Read the model definition and answer for the solid it produces. Units are mm, in the model's axes. A direction names the side the tool comes from. Coordinates: 2 decimals unless noted, no trailing zeros. Write each loop counter-clockwise with the first axis right and the second up, starting at its lowest first coordinate (ties: lowest second). Pieces come first, ordered by that corner, then holes.
(1) Given pin 1 (8 mm diameter, centred on y = 24, z = -23.74, fed in from -X); pin 2 (1.9 mm diameter, centred on x = -8.5, z = -22, fed in from +Y); pin 3 (1.9 mm diameter, centred on x = -7, z = -15, fed in from -Y), each flat-ended and moving along its own axis, determine where each tip first touches the part or whether it passes through.
(2) The mould has two halves that part along Z. Classify faces 4 (the cylindrical face through (-27.285, -1.521, -21.97)), 5 (the flat face through (-55, 71, -31.213)), 6 (the flat face through (-65.2, 116, -16)): +Z half, -Z half, draft (parallel to the pull), parting line (faces both ways), or undercut.
(3) Section C-C on x = -24.5 is taken. Write down the section's boundary in (y, z), then the cut area to 3 significant figures.
(4) Section B-B on x = -33.5 is taken. Write down the section's boundary in (y, z).
(5) Section A-A on y = 112 is taken. Write down the section's boundary in (x, z).
(6) Find the intervals of material crossed by probe 1 along X at (y, z) = (103, -13); probe 2 along X at (y, z) = (8.5, -20); probe 3 along Y at (x, z) = (-12.5, -22), in increasing order.
(7) Which of the six approach directions +Z, -Z, +X, -X, +Y, -Y give full straight-line access (tool end or side, diameter ignored) to faces 1 (the flat face through (-55.6, 41, -16)), 2 (the cylindrical face through (-54.079, 21.793, -21.712)), 3 (the flat face through (-34, 0, -13))?
from build123d import *

# Parameters (mm, degrees)
SKETCH_1_W                       = 44.2
SKETCH_1_H                       = 30
SM_BASE_FLANGE_1_DEPTH           = 3
SM_EDGE_FLANGE_1_STRIP_W         = 13.4732
SM_EDGE_FLANGE_1_STRIP_H         = 3
SM_EDGE_FLANGE_1_STRIP_CUT_DEPTH = 30
SM_EDGE_FLANGE_1_DEPTH           = 30
SM_EDGE_FLANGE_2_STRIP_W         = 13.4732
SM_EDGE_FLANGE_2_STRIP_H         = 3
SM_EDGE_FLANGE_2_STRIP_CUT_DEPTH = 30
SM_EDGE_FLANGE_2_DEPTH           = 30
SM_EDGE_FLANGE_3_STRIP_W         = 13.4732
SM_EDGE_FLANGE_3_STRIP_H         = 3
SM_EDGE_FLANGE_3_STRIP_CUT_DEPTH = 30
SM_EDGE_FLANGE_3_DEPTH           = 30
SM_EDGE_FLANGE_4_STRIP_W         = 13.4732
SM_EDGE_FLANGE_4_STRIP_H         = 3
SM_EDGE_FLANGE_4_STRIP_CUT_DEPTH = 30
SM_EDGE_FLANGE_4_DEPTH           = 30
SM_EDGE_FLANGE_5_STRIP_W         = 13.4732
SM_EDGE_FLANGE_5_STRIP_H         = 3
SM_EDGE_FLANGE_5_STRIP_CUT_DEPTH = 30
SM_EDGE_FLANGE_5_DEPTH           = 30
SM_EDGE_FLANGE_6_STRIP_W         = 13.4732
SM_EDGE_FLANGE_6_STRIP_H         = 3
SM_EDGE_FLANGE_6_STRIP_CUT_DEPTH = 30
SM_EDGE_FLANGE_6_DEPTH           = 30
SKETCH_20_R                      = 6
SKETCH_20_R_2                    = 1.05
CUT_EXTRUDE_1_DEPTH              = 100
SKETCH_21_R                      = 3
SKETCH_21_R_2                    = 1.5
CUT_EXTRUDE_2_DEPTH              = 10
SKETCH_22_R                      = 3
CUT_EXTRUDE_3_DEPTH              = 66


# Sheet-metal steps are written as plain solids
with BuildPart() as part:
    # Sketch 1 → 基体-法兰1 (new body)
    with BuildSketch(Plane(origin=(0, 0, 0), x_dir=(1, 0, 0), z_dir=(0, 1, 0))):
        with Locations((-33.5, 16.21342484)):
            Rectangle(SKETCH_1_W, SKETCH_1_H)
    extrude(amount=-SM_BASE_FLANGE_1_DEPTH)

    # 边线-法兰1 strip (across the edge) → 边线-法兰1 strip cut (cut)
    with BuildSketch(Plane(origin=(-55.6, 0, -31.21342484), x_dir=(1, 0, 0), z_dir=(0, 0, 1))):
        with Locations((-3, -1.5)):
            Rectangle(SM_EDGE_FLANGE_1_STRIP_W, SM_EDGE_FLANGE_1_STRIP_H)
    extrude(amount=SM_EDGE_FLANGE_1_STRIP_CUT_DEPTH, mode=Mode.SUBTRACT)

    # 边线-法兰1 section (across the edge) → 边线-法兰1 (add)
    with BuildSketch(Plane(origin=(-55.6, 0, -31.21342484), x_dir=(1, 0, 0), z_dir=(0, 0, 1))):
        with BuildLine():
            Line((0, 0.7366), (0, 87))
            Line((0, 87), (3, 87))
            Line((3, 87), (3, 0.7366))
            ThreePointArc((3, 0.7366), (3.215745145, 0.215745145), (3.7366, 0))
            Line((3.7366, 0), (3.7366, -3))
            ThreePointArc((3.7366, -3), (1.094424801, -1.905575199), (0, 0.7366))
        make_face()
    extrude(amount=SM_EDGE_FLANGE_1_DEPTH)

    # 边线-法兰2 strip (across the edge) → 边线-法兰2 strip cut (cut)
    with BuildSketch(Plane(origin=(-11.4, 0, -1.21342484), x_dir=(-1, 0, 0), z_dir=(0, 0, -1))):
        with Locations((-3, -1.5)):
            Rectangle(SM_EDGE_FLANGE_2_STRIP_W, SM_EDGE_FLANGE_2_STRIP_H)
    extrude(amount=SM_EDGE_FLANGE_2_STRIP_CUT_DEPTH, mode=Mode.SUBTRACT)

    # 边线-法兰2 section (across the edge) → 边线-法兰2 (add)
    with BuildSketch(Plane(origin=(-11.4, 0, -1.21342484), x_dir=(-1, 0, 0), z_dir=(0, 0, -1))):
        with BuildLine():
            Line((0, 0.7366), (0, 87))
            Line((0, 87), (3, 87))
            Line((3, 87), (3, 0.7366))
            ThreePointArc((3, 0.7366), (3.215745145, 0.215745145), (3.7366, 0))
            Line((3.7366, 0), (3.7366, -3))
            ThreePointArc((3.7366, -3), (1.094424801, -1.905575199), (0, 0.7366))
        make_face()
    extrude(amount=SM_EDGE_FLANGE_2_DEPTH)

    # 边线-法兰3 strip (across the edge) → 边线-法兰3 strip cut (cut)
    with BuildSketch(Plane(origin=(-11.4, 87, -31.21342484), x_dir=(0, -1, 0), z_dir=(0, 0, 1))):
        with Locations((-3, -1.5)):
            Rectangle(SM_EDGE_FLANGE_3_STRIP_W, SM_EDGE_FLANGE_3_STRIP_H)
    extrude(amount=SM_EDGE_FLANGE_3_STRIP_CUT_DEPTH, mode=Mode.SUBTRACT)

    # 边线-法兰3 section (across the edge) → 边线-法兰3 (add)
    with BuildSketch(Plane(origin=(-11.4, 87, -31.21342484), x_dir=(0, -1, 0), z_dir=(0, 0, 1))):
        with BuildLine():
            Line((0, 0.7366), (0, 10.8))
            Line((0, 10.8), (3, 10.8))
            Line((3, 10.8), (3, 0.7366))
            ThreePointArc((3, 0.7366), (3.215745145, 0.215745145), (3.7366, 0))
            Line((3.7366, 0), (3.7366, -3))
            ThreePointArc((3.7366, -3), (1.094424801, -1.905575199), (0, 0.7366))
        make_face()
    extrude(amount=SM_EDGE_FLANGE_3_DEPTH)

    # 边线-法兰4 strip (across the edge) → 边线-法兰4 strip cut (cut)
    with BuildSketch(Plane(origin=(-55.6, 87, -1.21342484), x_dir=(0, -1, 0), z_dir=(0, 0, -1))):
        with Locations((-3, -1.5)):
            Rectangle(SM_EDGE_FLANGE_4_STRIP_W, SM_EDGE_FLANGE_4_STRIP_H)
    extrude(amount=SM_EDGE_FLANGE_4_STRIP_CUT_DEPTH, mode=Mode.SUBTRACT)

    # 边线-法兰4 section (across the edge) → 边线-法兰4 (add)
    with BuildSketch(Plane(origin=(-55.6, 87, -1.21342484), x_dir=(0, -1, 0), z_dir=(0, 0, -1))):
        with BuildLine():
            Line((0, 0.7366), (0, 12.6))
            Line((0, 12.6), (3, 12.6))
            Line((3, 12.6), (3, 0.7366))
            ThreePointArc((3, 0.7366), (3.215745145, 0.215745145), (3.7366, 0))
            Line((3.7366, 0), (3.7366, -3))
            ThreePointArc((3.7366, -3), (1.094424801, -1.905575199), (0, 0.7366))
        make_face()
    extrude(amount=SM_EDGE_FLANGE_4_DEPTH)

    # 边线-法兰5 strip (across the edge) → 边线-法兰5 strip cut (cut)
    with BuildSketch(Plane(origin=(-68.2, 87, -31.21342484), x_dir=(1, 0, 0), z_dir=(0, 0, 1))):
        with Locations((-3, -1.5)):
            Rectangle(SM_EDGE_FLANGE_5_STRIP_W, SM_EDGE_FLANGE_5_STRIP_H)
    extrude(amount=SM_EDGE_FLANGE_5_STRIP_CUT_DEPTH, mode=Mode.SUBTRACT)

    # 边线-法兰5 section (across the edge) → 边线-法兰5 (add)
    with BuildSketch(Plane(origin=(-68.2, 87, -31.21342484), x_dir=(1, 0, 0), z_dir=(0, 0, 1))):
        with BuildLine():
            Line((0, 0.7366), (0, 72))
            Line((0, 72), (3, 72))
            Line((3, 72), (3, 0.7366))
            ThreePointArc((3, 0.7366), (3.215745145, 0.215745145), (3.7366, 0))
            Line((3.7366, 0), (3.7366, -3))
            ThreePointArc((3.7366, -3), (1.094424801, -1.905575199), (0, 0.7366))
        make_face()
    extrude(amount=SM_EDGE_FLANGE_5_DEPTH)

    # 边线-法兰6 strip (across the edge) → 边线-法兰6 strip cut (cut)
    with BuildSketch(Plane(origin=(-0.6, 87, -1.21342484), x_dir=(-1, 0, 0), z_dir=(0, 0, -1))):
        with Locations((-3, -1.5)):
            Rectangle(SM_EDGE_FLANGE_6_STRIP_W, SM_EDGE_FLANGE_6_STRIP_H)
    extrude(amount=SM_EDGE_FLANGE_6_STRIP_CUT_DEPTH, mode=Mode.SUBTRACT)

    # 边线-法兰6 section (across the edge) → 边线-法兰6 (add)
    with BuildSketch(Plane(origin=(-0.6, 87, -1.21342484), x_dir=(-1, 0, 0), z_dir=(0, 0, -1))):
        with BuildLine():
            Line((0, 0.7366), (0, 72))
            Line((0, 72), (3, 72))
            Line((3, 72), (3, 0.7366))
            ThreePointArc((3, 0.7366), (3.215745145, 0.215745145), (3.7366, 0))
            Line((3.7366, 0), (3.7366, -3))
            ThreePointArc((3.7366, -3), (1.094424801, -1.905575199), (0, 0.7366))
        make_face()
    extrude(amount=SM_EDGE_FLANGE_6_DEPTH)

    # 草图20 → 切除-拉伸1 (cut)
    with BuildSketch(Plane(origin=(-0.6, 0, 0), x_dir=(0, 0, -1), z_dir=(1, 0, 0))):
        with Locations(Location((16.21342484, 144, 0), (0, 0, 90))):
            Circle(SKETCH_20_R)
        with Locations(Location((16.21342484, 156, 0), (0, 0, 90))):
            Circle(SKETCH_20_R_2)
        with BuildLine():
            ThreePointArc((1.21342484, 144), (5.606823122, 154.606601718), (16.21342484, 159))
            Line((16.21342484, 159), (1.21342484, 159))
            Line((1.21342484, 159), (1.21342484, 144))
        make_face()
        with BuildLine():
            Line((31.21342484, 159), (16.21342484, 159))
            ThreePointArc((16.21342484, 159), (26.820026558, 154.606601718), (31.21342484, 144))
            Line((31.21342484, 144), (31.21342484, 159))
        make_face()
        with Locations(Location((24.698706214, 152.485281374, 0), (0, 0, 90))):
            Circle(SKETCH_20_R_2)
        with Locations(Location((28.21342484, 144, 0), (0, 0, 90))):
            Circle(SKETCH_20_R_2)
        with Locations(Location((24.698706214, 135.514718626, 0), (0, 0, 90))):
            Circle(SKETCH_20_R_2)
        with Locations(Location((16.21342484, 132, 0), (0, 0, 90))):
            Circle(SKETCH_20_R_2)
        with Locations(Location((7.728143465, 135.514718626, 0), (0, 0, 90))):
            Circle(SKETCH_20_R_2)
        with Locations(Location((4.21342484, 144, 0), (0, 0, 90))):
            Circle(SKETCH_20_R_2)
        with Locations(Location((7.728143465, 152.485281374, 0), (0, 0, 90))):
            Circle(SKETCH_20_R_2)
    extrude(amount=-CUT_EXTRUDE_1_DEPTH, mode=Mode.SUBTRACT)

    # 草图21 → 切除-拉伸2 (cut)
    with BuildSketch(Plane.XZ.offset(3)):
        with Locations(Location((-33.5, -16.21342484, 0), (0, 0, 270))):
            Circle(SKETCH_21_R)
        with Locations(Location((-28.550252532, -11.263677371, 0), (0, 0, 270))):
            Circle(SKETCH_21_R_2)
        with Locations(Location((-28.550252532, -21.163172308, 0), (0, 0, 270))):
            Circle(SKETCH_21_R_2)
        with Locations(Location((-38.449747468, -21.163172308, 0), (0, 0, 270))):
            Circle(SKETCH_21_R_2)
        with Locations(Location((-38.449747468, -11.263677371, 0), (0, 0, 270))):
            Circle(SKETCH_21_R_2)
    extrude(amount=-CUT_EXTRUDE_2_DEPTH, mode=Mode.SUBTRACT)

    # 草图22 → 切除-拉伸3 (cut)
    with BuildSketch(Plane(origin=(-11.4, 0, 0), x_dir=(0, 0, -1), z_dir=(1, 0, 0))):
        with BuildLine():
            ThreePointArc((10.708105598, 63.997198238), (7.293172758, 65.40967406), (8.709123695, 61.996180659))
            Line((8.709123695, 61.996180659), (8.708105857, 63.9961804))
            Line((8.708105857, 63.9961804), (10.708105598, 63.997198238))
        make_face()
        with BuildLine():
            Line((8.708105857, 63.9961804), (8.709123695, 61.996180659))
            ThreePointArc((8.709123695, 61.996180659), (10.122679234, 62.582326744), (10.708105857, 63.9961804))
            ThreePointArc((10.708105857, 63.9961804), (10.708105793, 63.996689319), (10.708105598, 63.997198238))
            Line((10.708105598, 63.997198238), (8.708105857, 63.9961804))
        make_face()
        with Locations(Location((23.739100582, 24.0038196, 0), (0, 0, 90))):
            Circle(SKETCH_22_R)
        with Locations(Location((8.72845873, 24.0038196, 0), (0, 0, 90))):
            Circle(SKETCH_22_R)
        with Locations(Location((23.718743822, 64.0038196, 0), (0, 0, 90))):
            Circle(SKETCH_22_R)
    extrude(amount=-CUT_EXTRUDE_3_DEPTH, mode=Mode.SUBTRACT)


solid = part.part
Response:
1. pin 1: stops at x = -55.6
1. pin 2: stops at y = 87
1. pin 3: stops at y = 84
2. face 4: undercut
2. face 5: -Z half
2. face 6: draft
3. outline: (-3, -31.21) - (0, -31.21) - (0, -1.21) - (-3, -1.21) - close
3. area: 90.0 mm2
4. outline: (-3, -31.21) - (0, -31.21) - (0, -19.21) - (-3, -19.21) - close; (-3, -13.21) - (0, -13.21) - (0, -1.21) - (-3, -1.21) - close
5. outline: (-68.2, -31.21) - (-65.2, -31.21) - (-65.2, -1.21) - (-68.2, -1.21) - close; (-3.6, -31.21) - (-0.6, -31.21) - (-0.6, -1.21) - (-3.6, -1.21) - close
6. probe 1: x = -68.2 to -65.2, -3.6 to -0.6
6. probe 2: x = -55.6 to -52.6, -14.4 to -11.4
6. probe 3: y = -1.91 to 21.56, 26.45 to 61.54, 66.46 to 86.52
7. face 1: +Z, -Z, -X, -Y
7. face 2: +X, -X
7. face 3: +Z, -Z, +Y
